```python
from build123d import *
from OCP.BRepFilletAPI import BRepFilletAPI_MakeChamfer

# Parameters (mm, degrees)
SKETCH_1_W                = 20
SKETCH_1_H                = 25
EXTRUDE_1_DEPTH           = 12.2
CUT_EXTRUDE_1_DEPTH       = 26.5
SKETCH_3_W                = 20
SKETCH_3_H                = 10
CUT_EXTRUDE_2_DEPTH       = 8.5
HOLE_WIZARD_1_D           = 3.2
HOLE_WIZARD_1_CSINK_D     = 6.1
HOLE_WIZARD_1_CSINK_ANGLE = 90
CHAMFER_1_SIZE            = 3
CHAMFER_1_SIZE2           = 1.03298284


with BuildPart() as part:
    # 草图1 → 凸台-拉伸1 (new body)
    with BuildSketch(Plane.XY):
        with Locations((117, 92.5)):
            Rectangle(SKETCH_1_W, SKETCH_1_H)
    extrude(amount=EXTRUDE_1_DEPTH)

    # 草图2 → 切除-拉伸1 (cut)
    with BuildSketch(Plane(origin=(0, 105, 0), x_dir=(1, 0, 0), z_dir=(0, 1, 0))):
        with BuildLine():
            Line((125.890619014, -7.895997518), (127, -3.195997518))
            Line((127, -3.195997518), (127, -12.2))
            Line((127, -12.2), (121.083012976, -12.2))
            ThreePointArc((121.083012976, -12.2), (124.162916731, -10.803208822), (125.890619014, -7.895997518))
        make_face()
    extrude(amount=-CUT_EXTRUDE_1_DEPTH, mode=Mode.SUBTRACT)

    # 草图3 → 切除-拉伸2 (cut)
    with BuildSketch(Plane.XY.offset(12.2)):
        with Locations((117, 92.5)):
            Rectangle(SKETCH_3_W, SKETCH_3_H)
    extrude(amount=-CUT_EXTRUDE_2_DEPTH, mode=Mode.SUBTRACT)

    # 打孔尺寸(%根据)内六角花形半沉头螺钉的类型1 (through all)
    with Locations(Plane.XY.offset(3.7)):
        with Locations((112, 92.5), (120, 92.5)):
            CounterSinkHole(HOLE_WIZARD_1_D / 2, HOLE_WIZARD_1_CSINK_D / 2, counter_sink_angle=HOLE_WIZARD_1_CSINK_ANGLE)

    # 倒角1: one chamfer whose edges measure the first distance from different faces: ONE call of the kernel's chamfer builder (chamfer() names one face for all edges)
    chamfer_1_edges_1 = [part.edges().sort_by_distance(p)[0] for p in [
        (116.940518003, 87.5, 3.7),
    ]]
    chamfer_1_side_1 = [part.faces().sort_by_distance(p)[0] for p in [
        (116.264670273, 87.5, 7.794514486),
    ]]
    chamfer_1_edges_2 = [part.edges().sort_by_distance(p)[0] for p in [
        (116.940518003, 97.5, 3.7),
    ]]
    chamfer_1_side_2 = [part.faces().sort_by_distance(p)[0] for p in [
        (116.264670273, 97.5, 7.794514486),
    ]]
    chamfer_1 = BRepFilletAPI_MakeChamfer(part.part.solid().wrapped)
    for e in chamfer_1_edges_1:
        chamfer_1.Add(CHAMFER_1_SIZE, CHAMFER_1_SIZE2, e.wrapped, chamfer_1_side_1[0].wrapped)  # the first distance lies on this face
    for e in chamfer_1_edges_2:
        chamfer_1.Add(CHAMFER_1_SIZE, CHAMFER_1_SIZE2, e.wrapped, chamfer_1_side_2[0].wrapped)  # the first distance lies on this face
    add(Compound.cast(chamfer_1.Shape()), mode=Mode.REPLACE)


solid = part.part
```
Input: part model. Units: mm. Frame: model coordinates. A direction names the side the tool comes from. Give positions to 0.01 mm unless a question says otherwise; leave off trailing zeros. Order: outer loops, then holes, each group sorted by start corner. A loop starts at its lowest first (then second) coordinate and runs counter-clockwise, first axis right, second up. Notation, with made-up numbers: (-31.75, -22) - (21.25, -22) arc R34 cw to (21.25, 11) - close; hole circle Ø4 at (14, 76). An arc over 180 degrees is marked (long way). Put each result on its own line as item: value.
Item 1: Section query B-B, the plane x = 120. Return loops of the section in (y, z).
Found:
outline: (80, 0) - (90.9, 0) - (90.9, 2.25) - (89.45, 3.7) - (88.53, 3.7) - (87.5, 6.7) - (87.5, 12.2) - (80, 12.2) - close; (94.1, 0) - (105, 0) - (105, 12.2) - (97.5, 12.2) - (97.5, 6.7) - (96.47, 3.7) - (95.55, 3.7) - (94.1, 2.25) - close
Item 2: Section query C-C, the plane z = 1.75. Return loops of the section in (x, y), then the cut area to 3 significant figures.
Found:
outline: (107, 80) - (127, 80) - (127, 105) - (107, 105) - close; hole circle Ø3.2 at (112, 92.5); hole circle Ø3.2 at (120, 92.5)
area: 484 mm^2
Item 3: Section query D-D, the plane z = 10.5. Return loops of the section in (x, y).
Found:
outline: (107, 80) - (124.48, 80) - (124.48, 87.5) - (107, 87.5) - close; (107, 97.5) - (124.48, 97.5) - (124.48, 105) - (107, 105) - close
Item 4: Access query for faces 1 (the cylindrical face through (110.474, 92.981, 1.109)), 2 (the flat face through (116, 97.5, 9)). Directions: +Z, -Z, +X, -X, +Y, -Y. A direction counts if a zero-diameter tool reaches every point of the face in a straight line with its end or side. Return the directions, or none.
Found:
face 1: +Z, -Z
face 2: +Z, +X, -X
Item 5: Ray query, L1, parallel to X at y = 92.5, z = 1.3; L2, parallel to Y at x = 109.25, z = 8.75; L3, parallel to Y at x = 112, z = 1.6. Return the intervals inside material, ascending. Write a range as from..to.
Found:
L1: x = 107..110.4, 113.6..118.4, 121.6..127
L2: y = 80..87.5, 97.5..105
L3: y = 80..90.9, 94.1..105
Item 6: Section query A-A, the plane y = 92.5. Return loops of the section in (x, z), then the cut area to 3 significant figures.
Found:
outline: (107, 0) - (110.4, 0) - (110.4, 2.25) - (108.95, 3.7) - (107, 3.7) - close; (113.6, 0) - (118.4, 0) - (118.4, 2.25) - (116.95, 3.7) - (115.05, 3.7) - (113.6, 2.25) - close; (121.6, 0) - (127, 0) - (127, 3.2) - (126.88, 3.7) - (123.05, 3.7) - (121.6, 2.25) - close
area: 46.1 mm^2
Item 7: Contact query for flat-ended pins moving along their axis: pin 1 (3.5 mm diameter, centred on x = 120, y = 92.5, fed in from +Z); pin 2 (1 mm diameter, centred on x = 124, y = 96, fed in from -Z); pin 3 (2 mm diameter, centred on y = 102, z = 8.5, fed in from +X); pin 4 (4 mm diameter, centred on x = 114.5, y = 94, fed in from +Z). Output: stop coordinate, or through.
Found:
pin 1: stops at z = 2.4
pin 2: stops at z = 0
pin 3: stops at x = 125.98
pin 4: stops at z = 3.7
Item 8: Draft query along Y for faces 3 (the flat face through (117, 105, 6)), 4 (the cylindrical face through (124.127, 83.803, 10.835)), 5 (the flat face through (116, 87.5, 9)). Return one class per face: +Y half, -Y half, draft (parallel to the pull), parting line (faces both ways), or undercut.
Found:
face 3: +Y half
face 4: draft
face 5: undercut
